Read the model definition and answer for the solid it produces. Units are mm, in the model's axes. Coordinates: 2 decimals unless noted, no trailing zeros. Loops run counter-clockwise (first coordinate to the right, second up) from the corner with the lowest first, then second, coordinate; pieces in that order, holes last. Notation, with made-up numbers: (-12, -18.75) -> (-1, -18.75) arc R8 cw to (-1, -8.75) -> close; hole circle Ø9 at (74, -5). An arc over 180 degrees is marked (long way). Answer as a JSON object with one key per item and string values. Group by question number.
Q1. Straight lines are drawn through the part: line 1 along Z through (x, y) = (75, -2.25); line 2 along Z through (x, y) = (233.5, 2); line 3 along Y through (x, z) = (68, 4.25). For each, find the intervals that lie inside material, in ascending order. Write a range as [from, to].
Q2. Each of these flat-tipped pins is pushed along its axis until it touches: P1, Ø1, axis at x = -188, z = 5.5, coming from the -Y side; P2, Ø6, axis at x = -89, y = -4, coming from the -Z side (3 decimals); P3, Ø4, axis at x = -0.5, y = 2, coming from the -Z side (3 decimals). Where does it stop, or does it pass through?
Q3. The part is cut by section B-B on y = 3.5. Write down the section's boundary in (x, z), and give its area (3 significant figures).
from build123d import *

# Parameters (mm, degrees)
BOSS_EXTRUDE1_DEPTH = 285.75


with BuildPart() as part:
    # Sketch1 → Boss-Extrude1 (new, symmetric)
    with BuildSketch(Plane(origin=(0, 0, 0), x_dir=(0, 0, -1), z_dir=(1, 0, 0))):
        with BuildLine():
            Line((7.188010851, 0.25), (3.810511777, 6.1))
            ThreePointArc((3.810511777, 6.1), (3.627499075, 6.283012702), (3.377499075, 6.35))
            Line((3.377499075, 6.35), (-3.377499075, 6.35))
            ThreePointArc((-3.377499075, 6.35), (-3.627499075, 6.283012702), (-3.810511777, 6.1))
            Line((-3.810511777, 6.1), (-7.188010851, 0.25))
            ThreePointArc((-7.188010851, 0.25), (-7.25499815, 0), (-7.188010851, -0.25))
            Line((-7.188010851, -0.25), (-3.810511777, -6.1))
            ThreePointArc((-3.810511777, -6.1), (-3.627499075, -6.283012702), (-3.377499075, -6.35))
            Line((-3.377499075, -6.35), (3.377499075, -6.35))
            ThreePointArc((3.377499075, -6.35), (3.627499075, -6.283012702), (3.810511777, -6.1))
            Line((3.810511777, -6.1), (7.188010851, -0.25))
            ThreePointArc((7.188010851, -0.25), (7.25499815, 0), (7.188010851, 0.25))
        make_face()
    extrude(amount=BOSS_EXTRUDE1_DEPTH, both=True)


solid = part.part
Final values:
{
 "1": {"line 1": "z = [-6.03, 6.03]", "line 2": "z = [-6.18, 6.18]", "line 3": "y = [-5.34, 5.34]"},
 "2": {"P1": "stops at y = -4.04", "P2": "stops at z = -6.755", "P3": "stops at z = -7.255"},
 "3": {"outline": "(-285.75, -5.31) -> (285.75, -5.31) -> (285.75, 5.31) -> (-285.75, 5.31) -> close", "area": "6,070 mm2"}
}
